Build history of the part. All positions in model axes, mm. Face numbers are marked on the shaded views. A direction names the side the tool comes from. Give positions to 0.01 mm unless a question says otherwise; leave off trailing zeros. Loops run counter-clockwise (first coordinate to the right, second up) from the corner with the lowest first, then second, coordinate; pieces in that order, holes last.
1) Band-saw the part on B-B on y = 0. List the corners of the cut face in (x, z) (1 decimal).
2) 3-axis set-ups, long thin cutter, end or side, ignore diameter. For the marked faces 5 and 6: which of +Z, -Z, +X, -X, +Y, -Y reach the whole face in a straight line?
3) Band-saw the part on C-C on z = 7. List the corners of the cut face in (x, y), then the cut area to 3 significant figures.
4) Band-saw the part on A-A on x = 0. List the corners of the cut face in (y, z) (1 decimal), then the cut area to 3 significant figures.
5) Two-plate mould, pull along X, no slides. Class the marked faces 1, 2, 3 and 4: +X half, -X half, draft (parallel to the pull), parting line (faces both ways), or undercut.
6) Wall check: line 1 (Y direction, x = 0, z = 16.5) (3 decimals); line 2 (X direction, y = -6, z = 3.25); line 3 (X direction, y = -13, z = 1.5). Give the ranges that are in metal, low to high.
7) Band-saw the part on D-D on z = 15.5. List the corners of the cut face in (x, y) (3 decimals).
8) Flat gauge pins, fed straight in: P1, Ø1, axis at y = -15, z = 5.5, coming from the -X side; P2, Ø1, axis at x = -18.5, z = 9, coming from the -Y side; P3, Ø2, axis at y = -2.5, z = 22.5, coming from the +X side; P4, Ø4, axis at x = 0, y = 0, coming from the -Z side. Where does each tip first touch, or does it go through?
```python
from build123d import *

# Parameters (mm, degrees)
F0_R     = 49.406354
F1_DEPTH = 25.4
F3_D     = 6.35
F4_W     = 34.925
F4_H     = 60.325
F5_DEPTH = 12.7
F6_R     = 5.08
F7_R     = 0.252521


with BuildPart() as f1:
    # F0 (on Top) → F1 (new body)
    with BuildSketch(Plane.XY):
        Circle(F0_R)
    extrude(amount=F1_DEPTH)

    # F3 (through all)
    with Locations(Plane.XY.offset(25.4)):
        with Locations((0, 0)):
            Hole(F3_D / 2)

    # F4 (on face) → F5 (cut)
    with BuildSketch(Plane(origin=(0, 0, 0), x_dir=(1, 0, 0), z_dir=(0, 0, -1))):
        Rectangle(F4_W, F4_H)
    extrude(amount=-F5_DEPTH, mode=Mode.SUBTRACT)

    # F6
    f6_edges = [f1.edges().sort_by_distance(p)[0] for p in [
        (-49.406354, 0, 25.4),
    ]]
    fillet(f6_edges, radius=F6_R)

    # F7
    f7_edges = [f1.edges().sort_by_distance(p)[0] for p in [
        (-17.4625, 30.1625, 6.35),
        (17.4625, 30.1625, 6.35),
        (-17.4625, -30.1625, 6.35),
        (17.4625, -30.1625, 6.35),
    ]]
    fillet(f7_edges, radius=F7_R)


solid = f1.part
```
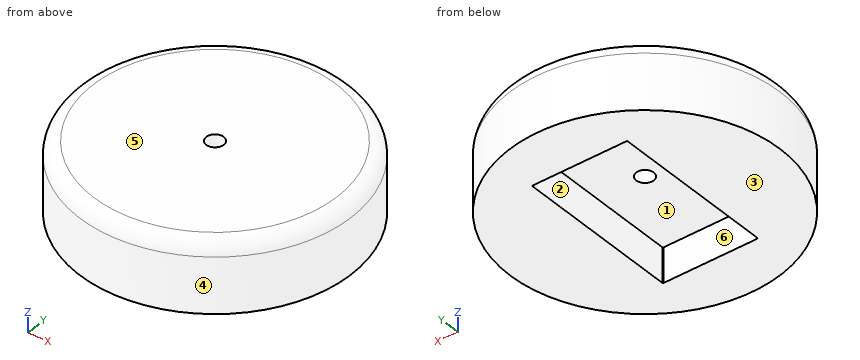
Findings below:
1. outline: (-49.4, 0) - (-17.5, 0) - (-17.5, 12.7) - (-3.2, 12.7) - (-3.2, 25.4) - (-44.3, 25.4) arc R5.1 ccw to (-49.4, 20.3) - close; (3.2, 12.7) - (17.5, 12.7) - (17.5, 0) - (49.4, 0) - (49.4, 20.3) arc R5.1 ccw to (44.3, 25.4) - (3.2, 25.4) - close
2. face 5: +Z, +X, -X, +Y, -Y
2. face 6: -Z
3. outline: circle Ø98.81 at (0, 0); hole (-17.46, -29.91) arc R0.25 ccw to (-17.21, -30.16) - (17.21, -30.16) arc R0.25 ccw to (17.46, -29.91) - (17.46, 29.91) arc R0.25 ccw to (17.21, 30.16) - (-17.21, 30.16) arc R0.25 ccw to (-17.46, 29.91) - close
3. area: 5,560 mm2
4. outline: (-49.4, 0) - (-30.2, 0) - (-30.2, 12.7) - (-3.2, 12.7) - (-3.2, 25.4) - (-44.3, 25.4) arc R5.1 ccw to (-49.4, 20.3) - close; (3.2, 12.7) - (30.2, 12.7) - (30.2, 0) - (49.4, 0) - (49.4, 20.3) arc R5.1 ccw to (44.3, 25.4) - (3.2, 25.4) - close
4. area: 1,650 mm2
5. face 1: undercut
5. face 2: undercut
5. face 3: draft
5. face 4: parting line
6. line 1: y = -49.406 to -3.175, 3.175 to 49.406
6. line 2: x = -49.04 to -17.46, 17.46 to 49.04
6. line 3: x = -47.67 to -17.46, 17.46 to 47.67
7. outline: circle Ø98.813 at (0, 0); hole circle Ø6.35 at (0, 0)
8. P1: stops at x = -47.23
8. P2: stops at y = -46.01
8. P3: stops at x = 49.21
8. P4: passes through
